```python
from build123d import *

# Parameters (mm, degrees)
SKETCH1_W           = 42.3
SKETCH1_H           = 42.3
BOSS_EXTRUDE1_DEPTH = 38
SKETCH2_R           = 11
BOSS_EXTRUDE2_DEPTH = 2
SKETCH3_R           = 2.5
BOSS_EXTRUDE4_DEPTH = 21.5
CUT_EXTRUDE1_START  = -18
CUT_EXTRUDE1_DEPTH  = 18
SKETCH5_R           = 1.55
CUT_EXTRUDE2_DEPTH  = 4.5
SKETCH6_OUTSIDE_W   = 61.46
SKETCH6_OUTSIDE_H   = 61.46
SKETCH6_OUTSIDE_W_2 = 42.3
SKETCH6_OUTSIDE_H_2 = 42.3
SKETCH6_OUTSIDE_R   = 1.55
CUT_EXTRUDE3_DEPTH  = 4.5


with BuildPart() as part:
    # Sketch1 → Boss-Extrude1 (new body)
    with BuildSketch(Plane.XY):
        with Locations((21.15, 21.15)):
            Rectangle(SKETCH1_W, SKETCH1_H)
    extrude(amount=BOSS_EXTRUDE1_DEPTH)

    # Sketch2 → Boss-Extrude2 (add)
    with BuildSketch(Plane.XY.offset(38)):
        with Locations((21.15, 21.15)):
            Circle(SKETCH2_R)
    extrude(amount=BOSS_EXTRUDE2_DEPTH)

    # Sketch3 → Boss-Extrude4 (add)
    with BuildSketch(Plane.XY.offset(40)):
        with Locations((21.15, 21.4)):
            Circle(SKETCH3_R)
    extrude(amount=BOSS_EXTRUDE4_DEPTH)

    # Sketch4 → Cut-Extrude1 (cut)
    with BuildSketch(Plane.XY.offset(61.5).offset(CUT_EXTRUDE1_START)):
        with BuildLine():
            Line((21.15, 23.4), (22.65, 23.4))
            ThreePointArc((22.65, 23.4), (21.15, 23.9), (19.65, 23.4))
            Line((19.65, 23.4), (21.15, 23.4))
        make_face()
    extrude(amount=CUT_EXTRUDE1_DEPTH, mode=Mode.SUBTRACT)

    # Sketch5 → Cut-Extrude2 (cut)
    with BuildSketch(Plane.XY.offset(38)):
        with Locations((5.65, 36.9)):
            Circle(SKETCH5_R)
        with Locations((36.65, 36.9)):
            Circle(SKETCH5_R)
        with Locations((36.65, 5.9)):
            Circle(SKETCH5_R)
        with Locations((5.65, 5.9)):
            Circle(SKETCH5_R)
    extrude(amount=-CUT_EXTRUDE2_DEPTH, mode=Mode.SUBTRACT)

    # Sketch6 outside → Cut-Extrude3 (cut)
    # profile 1 of 5: a face of its own
    with BuildSketch(Plane(origin=(0, 0, 0), x_dir=(-1, 0, 0), z_dir=(0, 0, -1))):
        with Locations((-21.15, 21.15)):
            Rectangle(SKETCH6_OUTSIDE_W, SKETCH6_OUTSIDE_H)
        with Locations((-21.15, 21.15)):
            Rectangle(SKETCH6_OUTSIDE_W_2, SKETCH6_OUTSIDE_H_2, mode=Mode.SUBTRACT)
    # profile 2 of 5: a face of its own
    with BuildSketch(Plane(origin=(0, 0, 0), x_dir=(-1, 0, 0), z_dir=(0, 0, -1))):
        with Locations(Location((-5.65, 36.9, 0), (0, 0, 180))):
            Circle(SKETCH6_OUTSIDE_R)
    # profile 3 of 5: a face of its own
    with BuildSketch(Plane(origin=(0, 0, 0), x_dir=(-1, 0, 0), z_dir=(0, 0, -1))):
        with Locations(Location((-36.65, 36.9, 0), (0, 0, 180))):
            Circle(SKETCH6_OUTSIDE_R)
    # profile 4 of 5: a face of its own
    with BuildSketch(Plane(origin=(0, 0, 0), x_dir=(-1, 0, 0), z_dir=(0, 0, -1))):
        with Locations(Location((-36.65, 5.9, 0), (0, 0, 180))):
            Circle(SKETCH6_OUTSIDE_R)
    # profile 5 of 5: a face of its own
    with BuildSketch(Plane(origin=(0, 0, 0), x_dir=(-1, 0, 0), z_dir=(0, 0, -1))):
        with Locations(Location((-5.65, 5.9, 0), (0, 0, 180))):
            Circle(SKETCH6_OUTSIDE_R)
    extrude(amount=-CUT_EXTRUDE3_DEPTH, mode=Mode.SUBTRACT)


solid = part.part
```
Input: part model. Units: mm. Frame: model coordinates. A direction names the side the tool comes from. Coordinates: 2 decimals unless noted, no trailing zeros. Write each loop counter-clockwise with the first axis right and the second up, starting at its lowest first coordinate (ties: lowest second). Pieces come first, ordered by that corner, then holes. Notation, with made-up numbers: (52, -7) -> (89, -7) arc R15 cw to (89, 3) -> close; hole circle Ø5 at (13.5, 65.25). An arc over 180 degrees is marked (long way). Answer as a JSON object with one key per item and string values.
1. Material intervals for line 1 (X direction, y = 36.9, z = 2.4); line 2 (Y direction, x = 36.65, z = 1); line 3 (Y direction, x = 7, z = 34), sorted ascending. Write a range as from..to.
Result set:
{"line 1": "x = 0..4.1, 7.2..35.1, 38.2..42.3", "line 2": "y = 0..4.35, 7.45..35.35, 38.45..42.3", "line 3": "y = 0..5.14, 6.66..36.14, 37.66..42.3"}
2. Section D-D on x = 5.65. Return the cut outline in (y, z), then the cut area to 3 significant figures.
Result set:
{"outline": "(0, 0) -> (4.35, 0) -> (4.35, 4.5) -> (7.45, 4.5) -> (7.45, 0) -> (35.35, 0) -> (35.35, 4.5) -> (38.45, 4.5) -> (38.45, 0) -> (42.3, 0) -> (42.3, 38) -> (38.45, 38) -> (38.45, 33.5) -> (35.35, 33.5) -> (35.35, 38) -> (7.45, 38) -> (7.45, 33.5) -> (4.35, 33.5) -> (4.35, 38) -> (0, 38) -> close", "area": "1,550 mm2"}
3. Section C-C on z = 55. Return the cut outline in (x, y), then the cut area to 3 significant figures.
Result set:
{"outline": "(19.65, 23.4) arc R2.5 ccw (long way) to (22.65, 23.4) -> close", "area": "18.6 mm2"}
4. First-contact query: P1, Ø1.5, axis at x = 37, y = 5.5, coming from the -Z side; P2, Ø3.5, axis at x = 37.5, y = 6, coming from the +Z side; P3, Ø6, axis at y = 18.5, z = 42.5, coming from the +X side. Flat tips, straight axial feed; report the tip coordinate or a pass-through.
Result set:
{"P1": "stops at z = 4.5", "P2": "stops at z = 38", "P3": "stops at x = 32.11"}
5. Section B-B on x = 21.15. Return the cut outline in (y, z), then the cut area to 3 significant figures.
Result set:
{"outline": "(0, 0) -> (42.3, 0) -> (42.3, 38) -> (32.15, 38) -> (32.15, 40) -> (23.9, 40) -> (23.9, 43.5) -> (23.4, 43.5) -> (23.4, 61.5) -> (18.9, 61.5) -> (18.9, 40) -> (10.15, 40) -> (10.15, 38) -> (0, 38) -> close", "area": "1,750 mm2"}
6. Access query for faces 4 (the face through (5.448, 35.363, 2.218)), 5 (the face through (21, 23.4, 52)), 6 (the face through (6, 6, 33.5)). Directions: +Z, -Z, +X, -X, +Y, -Y. A direction counts if a zero-diameter tool reaches every point of the face in a straight line with its end or side. Return the directions, or none.
Result set:
{"face 4": "-Z", "face 5": "+Z, +X, -X, +Y", "face 6": "+Z"}
7. Mould query, pull axis X, two halves, no side actions, for faces 1 (the face through (21, 42.3, 19)), 2 (the face through (13.04, 28.58, 38.99)), 3 (the face through (6, 37, 33.5)). Classes: released by +X, released by -X, zero draft, split by the parting line, or undercut.
Result set:
{"face 1": "zero draft", "face 2": "split by the parting line", "face 3": "undercut"}
8. Section A-A on y = 36.9. Return the cut outline in (x, z), then the cut area to 3 significant figures.
Result set:
{"outline": "(0, 0) -> (4.1, 0) -> (4.1, 4.5) -> (7.2, 4.5) -> (7.2, 0) -> (35.1, 0) -> (35.1, 4.5) -> (38.2, 4.5) -> (38.2, 0) -> (42.3, 0) -> (42.3, 38) -> (38.2, 38) -> (38.2, 33.5) -> (35.1, 33.5) -> (35.1, 38) -> (7.2, 38) -> (7.2, 33.5) -> (4.1, 33.5) -> (4.1, 38) -> (0, 38) -> close", "area": "1,550 mm2"}
